Can you work these out from the model? Positions are in its coordinate system, mm. A direction names the side the tool comes from. Coordinates: 2 decimals unless noted, no trailing zeros. Order: outer loops, then holes, each group sorted by start corner. A loop starts at its lowest first (then second) coordinate and runs counter-clockwise, first axis right, second up. Notation, with made-up numbers: (24, 69) - (34, 69) arc R15 ccw to (34, 76) - close; hole circle Ø11 at (17.25, 42). An arc over 180 degrees is marked (long way). Use a Markdown table: item, result. Add a question column.
(1) We'd pull the mould along X, two halves only. Please class faces 1 (the cylindrical face through (-17.859, 0.507, -14.797)), 2 (the cylindrical face through (17.797, 0.507, 14.859)), 3 (the cylindrical face through (-13.017, 0.493, -12.26)): pulls with the +X half, pulls with the -X half, needs draft (parallel to the pull), parting line crosses it, or undercut.
(2) For pin 1 Ø3 at (x, z) = (-15, -12) entering from +Y; pin 2 Ø9.5 at (x, z) = (-2, 2) entering from -Y; pin 3 Ø1.5 at (y, z) = (-1, -8.5) entering from -X, each with a flat end and sliding along its axis, tell me the tip position at first contact or that it passes through.
(3) On a 3-axis mill with a long thin cutter (end or side, diameter ignored), from which of +Z, -Z, +X, -X, +Y, -Y can I reach the whole of each face in a straight line? I mean faces 4 (the cylindrical face through (-7.91, -2.493, 10.316)), 5 (the flat face through (-0.2, 0.5, -16)). Say none if no direction works.
(4) If I drill on L1, parallel to X at y = 0.6, z = 12; L2, parallel to X at y = -0.45, z = -4; L3, parallel to Y at x = 16.5, z = 14, over which ranges is the centre line in solid material (lowest first)? Write a range as [from, to].
(5) I want a section at C-C (y = -0.5). List the corners of the cut face in (x, z) for me.
(6) I want a section at D-D (z = 12.5). State how many separate pieces and enclosed holes the cut face has, and give its area (3 significant figures).
```python
from build123d import *

# Parameters (mm, degrees)
SKETCH2_W           = 38
SKETCH2_H           = 32
SKETCH2_R           = 2
BOSS_EXTRUDE1_DEPTH = 1
FILLET1_R           = 4
SKETCH3_R           = 13
BOSS_EXTRUDE2_DEPTH = 3
SKETCH4_R           = 12
CUT_EXTRUDE1_DEPTH  = 2
FILLET2_R           = 2
SKETCH5_R           = 6
CUT_EXTRUDE4_DEPTH  = 1
SKETCH11_R          = 5
BOSS_EXTRUDE5_DEPTH = 2
FILLET7_R           = 1


with BuildPart() as part:
    # Sketch2 → Boss-Extrude1 (new body)
    with BuildSketch(Plane(origin=(0, 0, 0), x_dir=(1, 0, 0), z_dir=(0, 1, 0))):
        Rectangle(SKETCH2_W, SKETCH2_H)
        with Locations(Location((-15, 12, 0), (0, 0, 270))):
            Circle(SKETCH2_R, mode=Mode.SUBTRACT)
        with Locations(Location((15, 12, 0), (0, 0, 90))):
            Circle(SKETCH2_R, mode=Mode.SUBTRACT)
        with Locations(Location((15, -12, 0), (0, 0, 270))):
            Circle(SKETCH2_R, mode=Mode.SUBTRACT)
        with Locations(Location((-15, -12, 0), (0, 0, 90))):
            Circle(SKETCH2_R, mode=Mode.SUBTRACT)
    extrude(amount=BOSS_EXTRUDE1_DEPTH)

    # Fillet1
    fillet1_edges = [part.edges().sort_by_distance(p)[0] for p in [
        (-19, 0.5, -16),
        (19, 0.5, -16),
        (19, 0.5, 16),
        (-19, 0.5, 16),
    ]]
    fillet(fillet1_edges, radius=FILLET1_R)

    # Sketch3 → Boss-Extrude2 (add)
    with BuildSketch(Plane.XZ):
        with Locations(Location((0, 0, 0), (0, 0, 270))):
            Circle(SKETCH3_R)
    extrude(amount=BOSS_EXTRUDE2_DEPTH)

    # Sketch4 → Cut-Extrude1 (cut)
    with BuildSketch(Plane.XZ.offset(3)):
        with Locations(Location((0, 0, 0), (0, 0, 270))):
            Circle(SKETCH4_R)
    extrude(amount=-CUT_EXTRUDE1_DEPTH, mode=Mode.SUBTRACT)

    # Fillet2
    fillet2_edges = [part.edges().sort_by_distance(p)[0] for p in [
        (0, 0, 13),
    ]]
    fillet(fillet2_edges, radius=FILLET2_R)

    # Sketch5 → Cut-Extrude4 (cut)
    with BuildSketch(Plane.XZ.offset(1)):
        with Locations(Location((0, 0, 0), (0, 0, 270))):
            Circle(SKETCH5_R)
    extrude(amount=-CUT_EXTRUDE4_DEPTH, mode=Mode.SUBTRACT)

    # Sketch11 → Boss-Extrude5 (add)
    with BuildSketch(Plane.XZ):
        with Locations(Location((0, 0, 0), (0, 0, 270))):
            Circle(SKETCH11_R)
    extrude(amount=BOSS_EXTRUDE5_DEPTH)

    # Fillet7
    fillet7_edges = [part.edges().sort_by_distance(p)[0] for p in [
        (0, -1, 12),
        (0, -1, 6),
        (0, -2, 5),
    ]]
    fillet(fillet7_edges, radius=FILLET7_R - 0.0001)  # a hair under: the kernel refuses the full size


solid = part.part
```
Answers follow:
| question | item | result |
|---|---|---|
| 1 | face 1 | pulls with the -X half |
| 1 | face 2 | pulls with the +X half |
| 1 | face 3 | undercut |
| 2 | pin 1 | passes through |
| 2 | pin 2 | stops at y = -2 |
| 2 | pin 3 | stops at x = -11.26 |
| 3 | face 4 | -Y |
| 3 | face 5 | -Z, +X, -X, +Y, -Y |
| 4 | L1 | x = [-19, -17], [-13, 13], [17, 19] |
| 4 | L2 | x = [-13.14, -4.61], [-3, 3], [4.61, 13.14] |
| 4 | L3 | y = [0, 1] |
| 5 | outline | circle Ø27.35 at (0, 0); circle Ø10 at (0, 0); hole circle Ø12.27 at (0, 0) |
| 6 | separate pieces | 3 |
| 6 | enclosed holes | 0 |
| 6 | area | 56.5 mm² |
